Read the model definition and answer for the solid it produces. Units are mm, in the model's axes. Face numbers are marked on the shaded views. A direction names the side the tool comes from. Give positions to 0.01 mm unless a question says otherwise; leave off trailing zeros. Write each loop counter-clockwise with the first axis right and the second up, starting at its lowest first coordinate (ties: lowest second). Pieces come first, ordered by that corner, then holes. Notation, with made-up numbers: M 70.25,-39.75 L 98.25,-39.75 A23 cw 98.25,-25.75 Z; hole C 70,-3.75 d2. An arc over 180 degrees is marked long. Write each question's results on one line, items separated by ' | '. Start each with the question number.
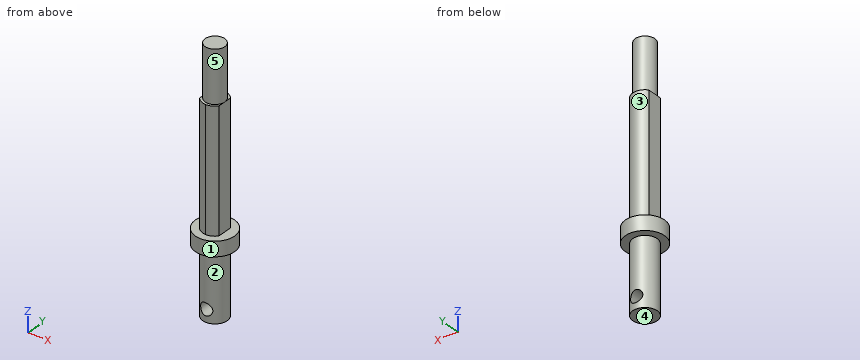
```python
from build123d import *

# Parameters (mm, degrees)
SKETCH1_R               = 2.5
BOSS_EXTRUDE1_DEPTH     = 13.8
BOSS_EXTRUDE3_START     = 13.8
SKETCH1_4_R             = 4
BOSS_EXTRUDE3_DEPTH     = 3
BOSS_EXTRUDE2_START     = 16.8
BOSS_EXTRUDE2_DEPTH     = 24.9
SKETCH2_R               = 2
BOSS_EXTRUDE4_DEPTH     = 10.6
SKETCH17_R              = 1.25
CUT_EXTRUDE1_DEPTH      = 53.605037782
CUT_EXTRUDE1_DEPTH_BACK = 53.605037782


with BuildPart() as part:
    # Sketch1 → Boss-Extrude1 (new body)
    with BuildSketch(Plane.XY):
        with Locations(Location((0, 0, 0), (0, 0, 180))):
            Circle(SKETCH1_R)
    extrude(amount=BOSS_EXTRUDE1_DEPTH)

    # Sketch1<4> → Boss-Extrude3 (add)
    with BuildSketch(Plane.XY.offset(BOSS_EXTRUDE3_START)):
        Circle(SKETCH1_4_R)
    extrude(amount=BOSS_EXTRUDE3_DEPTH)

    # Sketch1<3> → Boss-Extrude2 (add)
    with BuildSketch(Plane.XY.offset(BOSS_EXTRUDE2_START)):
        with BuildLine():
            ThreePointArc((0, -2.5), (1.099564058, -2.245207982), (1.975, -1.532767106))
            Line((1.975, -1.532767106), (1.975, 1.532767106))
            ThreePointArc((1.975, 1.532767106), (0, 2.5), (-1.975, 1.532767106))
            Line((-1.975, 1.532767106), (-1.975, -1.532767106))
            ThreePointArc((-1.975, -1.532767106), (-1.099564058, -2.245207982), (0, -2.5))
        make_face()
    extrude(amount=BOSS_EXTRUDE2_DEPTH)

    # Sketch2 → Boss-Extrude4 (add)
    with BuildSketch(Plane.XY.offset(41.7)):
        with Locations(Location((0, 0, 0), (0, 0, 170.931278454))):
            Circle(SKETCH2_R)
    extrude(amount=BOSS_EXTRUDE4_DEPTH)

    # Sketch17 → Cut-Extrude1 (cut, two sides)
    with BuildSketch(Plane(origin=(0, 0, 0), x_dir=(1, 0, 0), z_dir=(0, 1, 0))) as cut_extrude1_sk:
        with Locations(Location((0, -2.5, 0), (0, 0, 270))):
            Circle(SKETCH17_R)
    extrude(amount=CUT_EXTRUDE1_DEPTH, mode=Mode.SUBTRACT)
    extrude(cut_extrude1_sk.sketch, amount=-CUT_EXTRUDE1_DEPTH_BACK, mode=Mode.SUBTRACT)


solid = part.part
```
Item 1: Section C-C, the plane z = 2.5 is taken. Determine the outline of the cut face in (x, y), then the cut area to 3 significant figures.
Item 2: For the marked faces 1, 2, 3, 4 and 5, determine the directions among +Z, -Z, +X, -X, +Y, -Y from which every point of the face is accessible in a straight line to the end or side of a thin tool.
Item 3: Section B-B, the plane x = 3.5 is taken. Determine the outline of the cut face in (y, z), then the cut area to 3 significant figures.
Item 4: Section A-A, the plane z = 29 is taken. Determine the outline of the cut face in (x, y) (3 decimals).
Item 5: Section D-D, the plane y = -3 is taken. Determine the outline of the cut face in (x, z).
Item 6: Given P1, Ø4, axis at x = 0, z = 2.5, coming from the +Y side; P2, Ø2, axis at y = 2, z = 11.5, coming from the -X side; P3, Ø4, axis at y = -2, z = 9.5, coming from the +X side, each flat-ended and moving along its own axis, determine where each tip first touches the part or whether it passes through.
Item 7: Straight lines are drawn through the part: line 1 (Z direction, x = 0, y = -0.3); line 2 (X direction, y = 1, z = 27.5) (3 decimals); line 3 (X direction, y = -0.1, z = 2.5). For each, find the intervals that lie inside material, in ascending order.
Worked out:
1) outline: M -1.25,-2.17 L -1.25,2.17 A2.5 ccw Z; M 1.25,-2.17 A2.5 ccw 1.25,2.17 Z | area: 7.68 mm²
2) face 1: +Z, -Z | face 2: -Z | face 3: +Z, +Y | face 4: -Z, +X, -X, +Y, -Y | face 5: +Z
3) outline: M -1.94,13.8 L 1.94,13.8 L 1.94,16.8 L -1.94,16.8 Z | area: 11.6 mm²
4) outline: M -1.975,-1.533 A2.5 ccw 1.975,-1.533 L 1.975,1.533 A2.5 ccw -1.975,1.533 Z
5) outline: M -2.65,13.8 L 2.65,13.8 L 2.65,16.8 L -2.65,16.8 Z
6) P1: stops at y = 2.5 | P2: stops at x = -2.29 | P3: stops at x = 2.5
7) line 1: z = 0 to 1.25, 3.75 to 52.3 | line 2: x = -1.975 to 1.975 | line 3: x = -2.5 to -1.25, 1.25 to 2.5
